Could you check a few things on this model? Use its own coordinates, in mm. A direction names the side the tool comes from. Give positions to 0.01 mm unless a question says otherwise; leave off trailing zeros. Loops run counter-clockwise (first coordinate to the right, second up) from the corner with the lowest first, then second, coordinate; pieces in that order, holes last. Notation, with made-up numbers: (15, 31) -> (26, 31) arc R17 ccw to (26, 44) -> close; hole circle Ø11 at (-7, 78.25). An arc over 180 degrees is marked (long way). Put each result on its own line as item: value.
```python
from build123d import *

# Parameters (mm, degrees)
F0_W          = 22
F0_H          = 42
F1_DEPTH      = 3
F2_W          = 3
F2_H          = 30
F2_W_2        = 5
F3_DEPTH      = 22
F4_D          = 4.1
F7_DEPTH      = 5
F8_DEPTH      = 2.325
F9_R          = 4.99999
F11_D         = 4.1
F12_D         = 2.8
F13_W         = 22
F13_H         = 10.5
F14_DEPTH     = 8
F15_T1_DEPTH  = 8
F15_T3_DEPTH  = 18
F15_T5_DEPTH  = 18
F15_T7_DEPTH  = 22.7901994578
F15_T9_DEPTH  = 23
F15_T11_DEPTH = 23
F15_T13_DEPTH = 23
F16_D         = 29
F17_D         = 3.1


# Not quite as in the source:
# - a fillet or chamfer that OpenCascade refuses, or shapes differently, is made with other operations: its cross-section is extruded or revolved along the edge and cut away or added
# - a fillet or chamfer is up to 0.001 mm smaller than in the source, because OpenCascade refuses the exact size


with BuildPart() as f1:
    # F0 (on Front) → F1 (new body)
    with BuildSketch(Plane.XZ):
        with Locations((-28.9233987555, 27.9422005266)):
            Rectangle(F0_W, F0_H)
    extrude(amount=F1_DEPTH)

    # F2 (on face) → F3 (join)
    with BuildSketch(Plane(origin=(-39.9233987555, 0, 0), x_dir=(0, -1, 0), z_dir=(-1, 0, 0))):
        with Locations((1.5, 33.9422005266)):
            Rectangle(F2_W, F2_H)
        with Locations((5.5, 33.9422005266)):
            Rectangle(F2_W_2, F2_H)
    extrude(amount=-F3_DEPTH)

    # F4 (through all)
    with Locations(Plane(origin=(0, 0, 0), x_dir=(1, 0, 0), z_dir=(0, 1, 0))):
        with Locations((-24.9233987555, -12.9422005266), (-32.9233987555, -12.9422005266), (-32.9233987555, -32.9422005266), (-24.9233987555, -32.9422005266)):
            Hole(F4_D / 2)

    # F6 (on line) → F7 (join, symmetric)
    with BuildSketch(Plane.XY.offset(23.9422005266)):
        with BuildLine():
            ThreePointArc((-36.9233987555, -20), (-28.9233987555, -12), (-20.9233987555, -20))
            Line((-20.9233987555, -20), (-20.9233987555, -32))
            Line((-20.9233987555, -32), (-17.9233987555, -32))
            Line((-17.9233987555, -32), (-17.9233987555, 0))
            Line((-17.9233987555, 0), (-39.9233987555, 0))
            Line((-39.9233987555, 0), (-39.9233987555, -32))
            Line((-39.9233987555, -32), (-36.9233987555, -32))
            Line((-36.9233987555, -32), (-36.9233987555, -20))
        make_face()
    extrude(amount=F7_DEPTH, both=True)

    # F6 (on line) → F8 (join, symmetric)
    with BuildSketch(Plane.XY.offset(23.9422005266)):
        with BuildLine():
            ThreePointArc((-34.9233987555, -20), (-28.9233987555, -14), (-22.9233987555, -20))
            Line((-22.9233987555, -20), (-22.9233987555, -25.2915026221))
            ThreePointArc((-22.9233987555, -25.2915026221), (-21.4400839819, -22.8284271247), (-20.9233987555, -20))
            ThreePointArc((-20.9233987555, -20), (-28.9233987555, -12), (-36.9233987555, -20))
            ThreePointArc((-36.9233987555, -20), (-36.406713529, -22.8284271247), (-34.9233987555, -25.2915026221))
            Line((-34.9233987555, -25.2915026221), (-34.9233987555, -20))
        make_face()
        with BuildLine():
            Line((-34.9233987555, -32), (-34.9233987555, -25.2915026221))
            ThreePointArc((-34.9233987555, -25.2915026221), (-36.406713529, -22.8284271247), (-36.9233987555, -20))
            Line((-36.9233987555, -20), (-36.9233987555, -32))
            Line((-36.9233987555, -32), (-34.9233987555, -32))
        make_face()
        with BuildLine():
            ThreePointArc((-20.9233987555, -20), (-21.4400839819, -22.8284271247), (-22.9233987555, -25.2915026221))
            Line((-22.9233987555, -25.2915026221), (-22.9233987555, -32))
            Line((-22.9233987555, -32), (-20.9233987555, -32))
            Line((-20.9233987555, -32), (-20.9233987555, -20))
        make_face()
    extrude(amount=F8_DEPTH, both=True)

    # F9 (radius 5 in the source; OpenCascade refuses exactly that, so slightly less here)
    f9_edges = [f1.edges().sort_by_distance(p)[0] for p in [
        (-38.423399, -32, 28.942201),
        (-38.423399, -32, 18.942201),
        (-19.423399, -32, 18.942201),
        (-19.423399, -32, 28.942201),
    ]]
    fillet(f9_edges, radius=F9_R)

    # F11 (through all)
    with Locations(Plane(origin=(-39.9233987555, 0, 0), x_dir=(0, -1, 0), z_dir=(-1, 0, 0))):
        with Locations((4, 44.9422005266), (4, 24.9422005266)):
            Hole(F11_D / 2)

    # F12 (through all)
    with Locations(Plane(origin=(-39.9233987555, 0, 0), x_dir=(0, -1, 0), z_dir=(-1, 0, 0))):
        with Locations((27.5, 23.9422005266)):
            Hole(F12_D / 2)

    # F13 (on Front) → F14 (join)
    with BuildSketch(Plane.XZ):
        Polygon((-57.4233987555, 59.4422005266), (-39.9233987555, 59.4422005266), (-17.9233987555, 59.4422005266), (-15.4233987555, 59.4422005266), (-15.4233987555, 101.4422005266), (-57.4233987555, 101.4422005266), align=None)
        with Locations((-28.9233987555, 54.1922005266)):
            Rectangle(F13_W, F13_H)
    extrude(amount=F14_DEPTH)

    # F15: fillet of radius 3 on 7 edges, made by hand

    # F15_s2 → F15_t1 (join)
    with BuildSketch(Plane.XZ):
        with BuildLine():
            ThreePointArc((-39.9233987555, 56.4422005266), (-40.8020784119, 58.5635208702), (-42.9233987555, 59.4422005266))
            Line((-42.9233987555, 59.4422005266), (-39.9233987555, 59.4422005266))
            Line((-39.9233987555, 59.4422005266), (-39.9233987555, 56.4422005266))
        make_face()
    extrude(amount=F15_T1_DEPTH)

    # F15_s4 → F15_t3 (cut)
    with BuildSketch(Plane.XZ.offset(-7.5)):
        with BuildLine():
            ThreePointArc((-39.9233987555, 9.9422005266), (-39.0447190991, 7.820880183), (-36.9233987555, 6.9422005266))
            Line((-36.9233987555, 6.9422005266), (-39.9233987555, 6.9422005266))
            Line((-39.9233987555, 6.9422005266), (-39.9233987555, 9.9422005266))
        make_face()
    extrude(amount=F15_T3_DEPTH, mode=Mode.SUBTRACT)

    # F15_s6 → F15_t5 (cut)
    with BuildSketch(Plane.XZ.offset(-7.5)):
        with BuildLine():
            ThreePointArc((-17.9233987555, 9.9422005266), (-18.8020784119, 7.820880183), (-20.9233987555, 6.9422005266))
            Line((-20.9233987555, 6.9422005266), (-17.9233987555, 6.9422005266))
            Line((-17.9233987555, 6.9422005266), (-17.9233987555, 9.9422005266))
        make_face()
    extrude(amount=F15_T5_DEPTH, mode=Mode.SUBTRACT)

    # F15_s8 → F15_t7 (cut)
    with BuildSketch(Plane.XZ.offset(-7.3950997289)):
        with BuildLine():
            ThreePointArc((-17.9233987555, 59.4422005266), (-16.132110908, 60.463748745), (-15.4233987555, 62.4002404181))
            Line((-15.4233987555, 62.4002404181), (-15.4233987555, 59.4422005266))
            Line((-15.4233987555, 59.4422005266), (-17.9233987555, 59.4422005266))
        make_face()
    extrude(amount=F15_T7_DEPTH, mode=Mode.SUBTRACT)

    # F15_s10 → F15_t9 (cut)
    with BuildSketch(Plane.XZ.offset(-7.5)):
        with BuildLine():
            ThreePointArc((-18.4233987555, 101.4422005266), (-16.3020784119, 100.5635208702), (-15.4233987555, 98.4422005266))
            Line((-15.4233987555, 98.4422005266), (-15.4233987555, 101.4422005266))
            Line((-15.4233987555, 101.4422005266), (-18.4233987555, 101.4422005266))
        make_face()
    extrude(amount=F15_T9_DEPTH, mode=Mode.SUBTRACT)

    # F15_s12 → F15_t11 (cut)
    with BuildSketch(Plane.XZ.offset(-7.5)):
        with BuildLine():
            ThreePointArc((-57.4233987555, 98.4422005266), (-56.5447190991, 100.5635208702), (-54.4233987555, 101.4422005266))
            Line((-54.4233987555, 101.4422005266), (-57.4233987555, 101.4422005266))
            Line((-57.4233987555, 101.4422005266), (-57.4233987555, 98.4422005266))
        make_face()
    extrude(amount=F15_T11_DEPTH, mode=Mode.SUBTRACT)

    # F15_s14 → F15_t13 (cut)
    with BuildSketch(Plane.XZ.offset(-7.5)):
        with BuildLine():
            ThreePointArc((-54.4233987555, 59.4422005266), (-56.5447190991, 60.320880183), (-57.4233987555, 62.4422005266))
            Line((-57.4233987555, 62.4422005266), (-57.4233987555, 59.4422005266))
            Line((-57.4233987555, 59.4422005266), (-54.4233987555, 59.4422005266))
        make_face()
    extrude(amount=F15_T13_DEPTH, mode=Mode.SUBTRACT)

    # F16 (through all)
    with Locations(Plane(origin=(0, 0, 0), x_dir=(1, 0, 0), z_dir=(0, 1, 0))):
        with Locations((-36.4233987555, -80.4422005266)):
            Hole(F16_D / 2)

    # F17 (through all)
    with Locations(Plane(origin=(0, 0, 0), x_dir=(1, 0, 0), z_dir=(0, 1, 0))):
        with Locations((-51.9233987555, -95.9422005266), (-20.9233987555, -95.9422005266), (-20.9233987555, -64.9422005266), (-51.9233987555, -64.9422005266)):
            Hole(F17_D / 2)


solid = f1.part
```
1. If we section it at A-A (y = -21.5): List the corners of the cut face in (x, z) for me.
Recorded:
outline: (-39.92, 18.94) -> (-36.92, 18.94) -> (-36.92, 21.62) -> (-34.92, 21.62) -> (-34.92, 26.27) -> (-36.92, 26.27) -> (-36.92, 28.94) -> (-39.92, 28.94) -> close; (-22.92, 21.62) -> (-20.92, 21.62) -> (-20.92, 18.94) -> (-17.92, 18.94) -> (-17.92, 28.94) -> (-20.92, 28.94) -> (-20.92, 26.27) -> (-22.92, 26.27) -> close
2. If we section it at D-D (z = 36): List the corners of the cut face in (x, y) for me, then the cut area to 3 significant figures.
Recorded:
outline: (-39.92, -8) -> (-17.92, -8) -> (-17.92, 0) -> (-39.92, 0) -> close
area: 176 mm^2
3. If we section it at C-C (z = 87.5): List the corners of the cut face in (x, y) for me, then the cut area to 3 significant figures.
Recorded:
outline: (-57.42, -8) -> (-49.09, -8) -> (-49.09, 0) -> (-57.42, 0) -> close; (-23.76, -8) -> (-15.42, -8) -> (-15.42, 0) -> (-23.76, 0) -> close
area: 133 mm^2
4. If we section it at B-B (y = -4): Count the separate pieces of the cut face and the enclosed holes in it, then the cut area to 3 significant figures.
Recorded:
separate pieces: 3
enclosed holes: 7
area: 1,750 mm^2
5. Thinking about a two-plate mould opening in X: for faces 1 (the face through (-36, -4, 101.442)), 2 (the face through (-39.923, -12, 28)), 3 (the face through (-33, -15, 26.267)), which applies, pulls with the +X half, pulls with the -X half, needs draft (parallel to the pull), parting line crosses it, or undercut?
Recorded:
face 1: needs draft
face 2: pulls with the -X half
face 3: undercut
6. I need wall thicknesses on line 1 (Z direction, x = -34.75, y = -4); line 2 (Z direction, x = -32.5, y = -6.5); line 3 (Z direction, x = -31.5, y = -2.5). Which ranges of each line are inside material? Lowest first, please.
Recorded:
line 1: z = 18.94 to 22.89, 26.99 to 32.01, 33.87 to 42.89, 46.99 to 66.04, 94.85 to 101.44
line 2: z = 18.94 to 30.94, 34.95 to 66.48, 94.4 to 101.44
line 3: z = 6.94 to 11.47, 14.42 to 23.54, 26.34 to 31.47, 34.42 to 43.54, 46.34 to 66.8, 94.08 to 101.44
7. I'm going to push flat-ended pins straight in: pin 1 (17.5 mm diameter, centred on x = -31.5, y = -12.5, fed in from -Z); pin 2 (6 mm diameter, centred on y = -10, z = 43.5, fed in from +X); pin 3 (4 mm diameter, centred on x = -20.92, z = 64.94, fed in from -Y). Where does each tip first touch, or does it pass through?
Recorded:
pin 1: stops at z = 18.94
pin 2: stops at x = -17.92
pin 3: stops at y = -8
8. For faces 4 (the face through (-36.923, -26, 28)), 5 (the face through (-36.1, -8, 65.7)), 6 (the face through (-49, -4, 59.442)), which set-ups out of +Z, -Z, +X, -X, +Y, -Y let a thin tool reach every point of the face, with its end or its side?
Recorded:
face 4: +Z, -Y
face 5: +Z, +X, -X, -Y
face 6: -Z, -X, +Y, -Y
